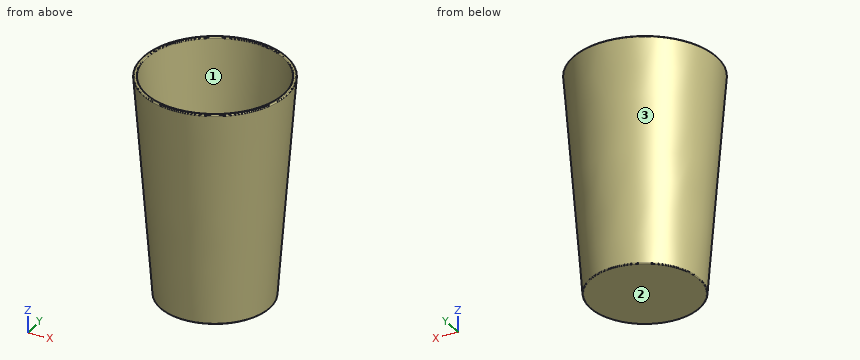
from build123d import *

# Parameters (mm, degrees)
F2_R = 0.396875
F3_R = 0.396875
F4_R = 0.396875


with BuildPart() as f1:
    # F0 (on Front) → F1 (revolve)
    with BuildSketch(Plane.XZ):
        Polygon((0, 1.5875), (0, 0), (25.4, 0), (33.3375, 101.6), (31.75, 101.6), (23.936523, 1.5875), align=None)
    revolve(axis=Axis((0, 0, 50.8), (0, 0, 1)))

    # F2
    f2_edges = [f1.edges().sort_by_distance(p)[0] for p in [
        (-33.3375, 0, 101.6),
    ]]
    fillet(f2_edges, radius=F2_R)

    # F3
    f3_edges = [f1.edges().sort_by_distance(p)[0] for p in [
        (-31.75, 0, 101.6),
    ]]
    fillet(f3_edges, radius=F3_R)

    # F4
    f4_edges = [f1.edges().sort_by_distance(p)[0] for p in [
        (-25.4, 0, 0),
    ]]
    fillet(f4_edges, radius=F4_R)


solid = f1.part
For this review, take the finished solid that the model builds, in its own axes (mm). Face numbers are marked on the shaded views. Round coordinates to 2 decimals unless told otherwise and drop trailing zeros. Loops run counter-clockwise (first coordinate to the right, second up) from the corner with the lowest first, then second, coordinate; pieces in that order, holes last. Notation, with made-up numbers: (76.5, 8.5) - (109.5, 8.5) arc R23 ccw to (109.5, 43.5) - close; hole circle Ø4 at (27.5, 78). An arc over 180 degrees is marked (long way). Put each result on its own line as item: value. Start each with the question number.
1. For probe 1 along Z at (x, y) = (-13.5, 16.5); probe 2 along X at (y, z) = (-6, 49); probe 3 along Y at (x, z) = (20.5, 63), list the stretches that pass through material, from the lowest coordinate up. Write a range as [from, to].
2. Consider section D-D on z = 95. State the section outline as (x, y) points.
3. Consider section A-A on y = 0. State the section outline as (x, z) points, plus the area to 3 significant figures.
4. Insertion check: P1, Ø12, axis at x = -8.5, z = 64, coming from the +Y side; P2, Ø10, axis at x = -11.5, z = 85.5, coming from the -Y side; P3, Ø2, axis at x = 11, z = 45, coming from the -Y side. Each pin has a flat end and moves straight along its axis. Give the tip position at first contact, or say it passes through.
5. Mouldability with a two-part tool opening along X and no side actions: class the marked faces 1, 2 and 3 as +X half, -X half, draft (parallel to the pull), parting line (faces both ways), or undercut.
6. Consider section C-C on z = 27. State the section outline as (x, y) points, plus the area to 3 significant figures.
Result sheet:
1. probe 1: [0, 1.59]
1. probe 2: [-28.61, -26.98], [26.98, 28.61]
1. probe 3: [-22.34, -20.13], [20.13, 22.34]
2. outline: circle Ø65.64 at (0, 0); hole circle Ø62.47 at (0, 0)
3. outline: (-33.3, 101.17) - (-25.43, 0.37) arc R0.4 ccw to (-25.03, 0) - (25.03, 0) arc R0.4 ccw to (25.43, 0.37) - (33.3, 101.17) arc R0.4 ccw to (32.91, 101.6) - (32.12, 101.6) arc R0.4 ccw to (31.72, 101.23) - (23.94, 1.59) - (-23.94, 1.59) - (-31.72, 101.23) arc R0.4 ccw to (-32.12, 101.6) - (-32.91, 101.6) arc R0.4 ccw to start
3. area: 398 mm^2
4. P1: y = 30.46
4. P2: y = -31.49
4. P3: y = -27.14
5. face 1: undercut
5. face 2: draft
5. face 3: parting line
6. outline: circle Ø55.02 at (0, 0); hole circle Ø51.84 at (0, 0)
6. area: 266 mm^2
